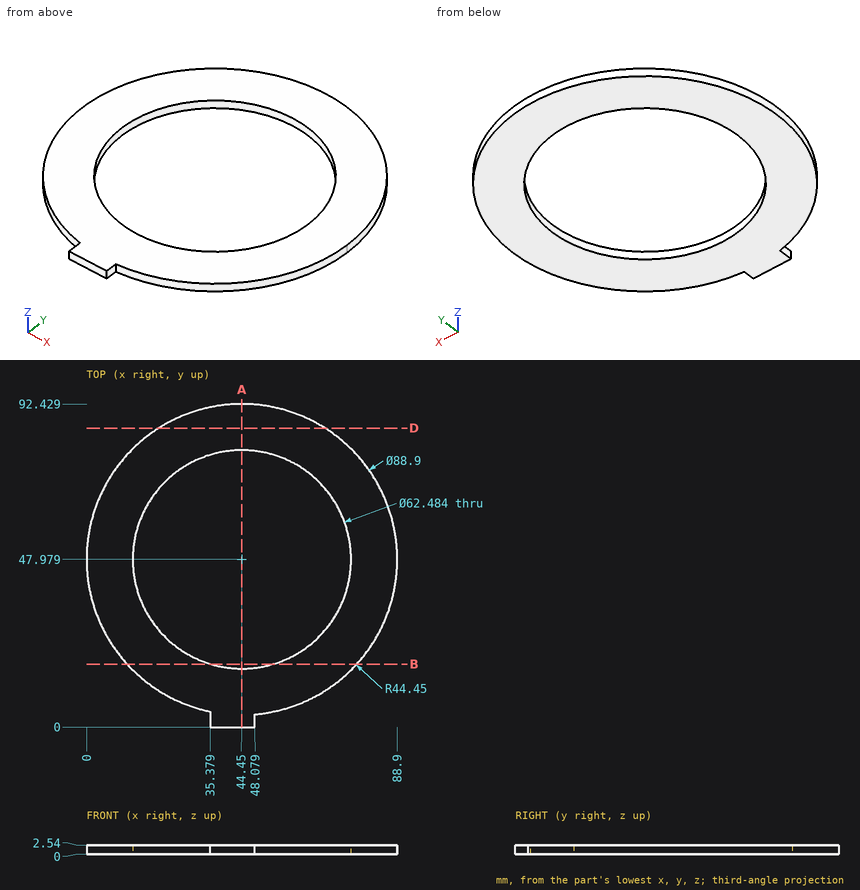
Geometry check sheet. Reference: drawing and pictorial views, mm from the part's lowest x, y, z. Round coordinates to 2 decimals unless told otherwise and drop trailing zeros. Loops run counter-clockwise (first coordinate to the right, second up) from the corner with the lowest first, then second, coordinate; pieces in that order, holes last. Notation, with made-up numbers: M -38.75,-5 L 11.25,-5 A14 cw 11.25,3 Z; hole C -28.75,34.25 d1. An arc over 180 degrees is marked long. One line per item, written item: value.
(1) Sectioned sample at D-D, the plane y = 85.5. Record the cut outline in (x, z), then the cut area to 3 significant figures.
Computed values:
outline: M 20.62,0 L 68.28,0 L 68.28,2.54 L 20.62,2.54 Z
area: 121 mm^2
(2) Sectioned sample at B-B, the plane y = 18. Record the cut outline in (x, z).
Computed values:
outline: M 11.63,0 L 35.66,0 L 35.66,2.54 L 11.63,2.54 Z; M 53.24,0 L 77.27,0 L 77.27,2.54 L 53.24,2.54 Z
(3) Sectioned sample at A-A, the plane x = 44.45. Record the cut outline in (y, z).
Computed values:
outline: M 0,0 L 16.74,0 L 16.74,2.54 L 0,2.54 Z; M 79.22,0 L 92.43,0 L 92.43,2.54 L 79.22,2.54 Z
(4) Depth check by flat-ended pin: pin 1 Ø1 at (y, z) = (30.5, 1) entering from -X; pin 2 Ø1.3 at (y, z) = (1, 1.5) entering from +X; pin 3 Ø1 at (x, y) = (36.5, 76.5) entering from +Z. Enter the tip coordinate at first touch or a pass-through.
Computed values:
pin 1: stops at x = 3.37
pin 2: stops at x = 48.08
pin 3: passes through
(5) Thickness scan on line 1 (Y direction, x = 44.45, z = 0.8); line 2 (X direction, y = 35, z = 0.7); line 3 (X direction, y = 39.5, z = 0.9) (1 decimal). Record the ranges inside material, lowest first.
Computed values:
line 1: y = 0 to 16.74, 79.22 to 92.43
line 2: x = 1.94 to 16.03, 72.87 to 86.96
line 3: x = 0.8 to 14.4, 74.5 to 88.1
